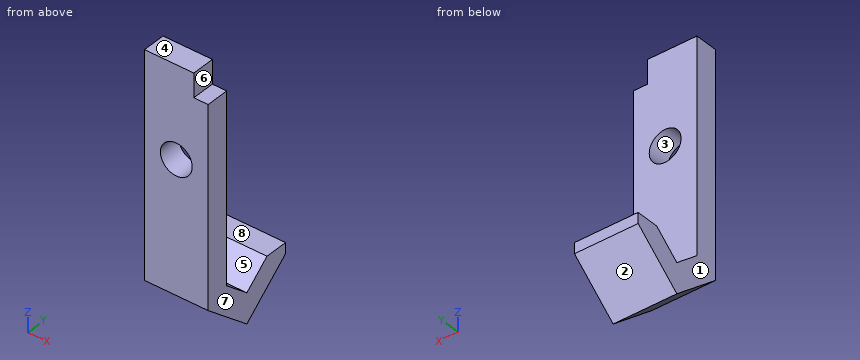
Autodesk Inventor part; units mm, degrees
ref_plane "YZ Plane" through (0, 0, 0) normal (1, 0, 0) x (0, 1, 0)
ref_plane "XZ Plane" through (0, 0, 0) normal (0, 1, 0) x (-1, 0, 0)
ref_plane "XY Plane" through (0, 0, 0) normal (0, 0, 1) x (1, 0, 0)
sketch "Sketch1" plane through (0, 0, 0) normal (1, 0, 0) x (0, 1, 0)
  line L0 (0, 0) -> (2.9, 0)
  line L1 (2.9, 0) -> (2.9, -25)
  line L2 (2.9, -25) -> (0, -25)
  line L3 (0, -25) -> (0, 0)
  line L4 (0, -25) -> (6.05, -30.0766)
  line L5 (2.9, -23.6477) -> (6.05, -26.2909)
  line L6 (6.05, -30.0766) -> (6.05, -26.2909)
  line L7 (6.05, -26.2909) -> (9.2, -23.6477)
  line L8 (6.05, -30.0766) -> (12.1, -25)
  line L9 (9.2, -27.4334) -> (9.2, -23.6477)
  line L10 (7.5884, -25) -> (12.1, -25)
  line L11 (12.1, -25) -> (12.1, -23.6477)
  line L12 (12.1, -23.6477) -> (9.2, -23.6477)
  dimension "d0" = 2.9
  dimension "d1" = 25
  dimension "d2" = 50
  dimension "d3" = 3.15
  dimension "d4" = 2.9
  dimension "d5" = 50
  dimension "d6" = 3.15
extrude "Extrusion1" add sketch "Sketch1" along normal blind 8
sketch "Sketch2" plane through (0, 0, 0) normal (0, 0, 1) x (1, 0, 0)
  line L0 (0, 0) -> (8, 0)
  line L1 (0, 0) -> (6.2, 0)
  line L2 (6.2, 0) -> (6.2, 2.9)
  line L3 (6.2, 2.9) -> (0, 2.9)
  line L4 (0, 2.9) -> (0, 0)
  dimension "d11" = 6.2
extrude "Extrusion2" add sketch "Sketch2" along normal blind 3
sketch "Sketch3" plane through (0, 2.9, -23.6477) normal (0, 1, 0) x (1, 0, 0)
  line L0 (6.2, -23.6477) -> (8, -23.6477)
  line L1 (0, -23.6477) -> (8, -23.6477)
  line L2 (4, -23.6477) -> (4, -15.1477)
  circle A0 centre (4, -15.1477) radius 2
  dimension "d14" = 8.5
  dimension "d15" = 4
extrude "Extrusion3" cut sketch "Sketch3" against normal through all
equation "\"d6\" = d3"
properties part number "Cap Pulley Support V2 Pt1" material "Thermoplastic Resin"
The model under review builds one solid part; all positions refer to its coordinate system, in mm. Face numbers are marked on the shaded views. A direction names the side the tool comes from. Round coordinates to 2 decimals unless told otherwise and drop trailing zeros. Order: outer loops, then holes, each group sorted by start corner. A loop starts at its lowest first (then second) coordinate and runs counter-clockwise, first axis right, second up. Notation, with made-up numbers: (-19.5, 29) -> (17.5, 29) arc R28 cw to (17.5, 65) -> close; hole circle Ø9 at (66, 22). An arc over 180 degrees is marked (long way). One line per item, written item: value. Start each with the question number.
Q1. Machinability: for the marked faces 5, 6, 7 and 8, which of the approach directions +Z, -Z, +X, -X, +Y, -Y give a long, thin tool a straight path to every point of the face, cutting with its end or side? Answer none if there is none.
Q2. Clearance check with flat-ended pins moving along their axes: pin 1 Ø2 at (x, y) = (4, 2.5) entering from -Z; pin 2 Ø3 at (y, z) = (3.5, -4.5) entering from +X; pin 3 Ø0.9 at (x, y) = (2, 10.5) entering from +Z; pin 4 Ø1 at (x, y) = (3, 10.5) entering from -Z. State where each tip first meets the part, or that it passes through.
Q3. Mouldability with a two-part tool opening along Z and no side actions: class the marked faces 1, 2, 3 and 4 as released by +Z, released by -Z, zero draft, split by the parting line, or undercut.
Q4. Take a section at A-A (x = 4). Write out the cut boundary in (y, z).
Q5. Take a section at C-C (x = 1.25). Write out the cut boundary in (y, z).
Q6. Take a section at B-B (z = -8.5). Write out the cut boundary in (x, y), and give its area (3 significant figures).
Q7. Take a section at D-D (z = -2). Write out the cut boundary in (x, y), and give its area (3 significant figures).
Q8. Wall thickness on line 1 (X direction, y = 0.7, z = -8.5); line 2 (Y direction, x = 2, z = -19); line 3 (Z direction, x = 4, y = 1.7): over which ranges is each line inside the solid? List them lowest first.
Reported:
1. face 5: +Z, +X, -X
1. face 6: +Z, +X, +Y, -Y
1. face 7: +Z, -Z, +X, +Y, -Y
1. face 8: +Z, +X, -X, +Y
2. pin 1: stops at z = -27.94
2. pin 2: stops at x = 8
2. pin 3: stops at z = -23.65
2. pin 4: stops at z = -26.76
3. face 1: zero draft
3. face 2: released by -Z
3. face 3: undercut
3. face 4: released by +Z
4. outline: (0, -25) -> (6.05, -30.08) -> (12.1, -25) -> (12.1, -23.65) -> (9.2, -23.65) -> (6.05, -26.29) -> (2.9, -23.65) -> (2.9, -10.5) -> (0, -10.5) -> close; (0, -6.5) -> (2.9, -6.5) -> (2.9, 3) -> (0, 3) -> close
5. outline: (0, -25) -> (6.05, -30.08) -> (12.1, -25) -> (12.1, -23.65) -> (9.2, -23.65) -> (6.05, -26.29) -> (2.9, -23.65) -> (2.9, 3) -> (0, 3) -> close
6. outline: (0, 0) -> (2, 0) -> (2, 2.9) -> (0, 2.9) -> close; (6, 0) -> (8, 0) -> (8, 2.9) -> (6, 2.9) -> close
6. area: 11.6 mm2
7. outline: (0, 0) -> (8, 0) -> (8, 2.9) -> (0, 2.9) -> close
7. area: 23.2 mm2
8. line 1: x = 0 to 2, 6 to 8
8. line 2: y = 0 to 2.9
8. line 3: z = -26.43 to -10.5, -6.5 to 3
